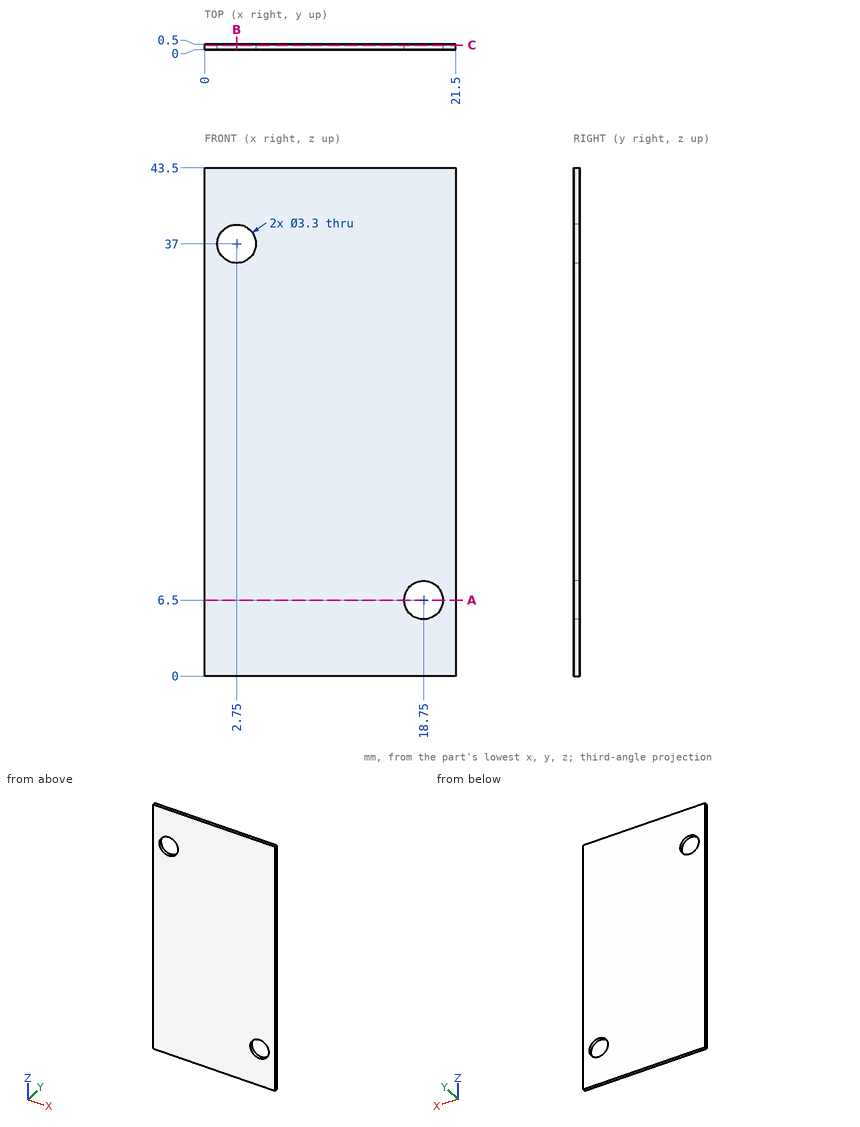
The drawing under review shows one solid part. Ordinate dimensions are in mm from its lowest x, y, z. Coordinates: 2 decimals unless noted, no trailing zeros. Write each loop counter-clockwise with the first axis right and the second up, starting at its lowest first coordinate (ties: lowest second). Pieces come first, ordered by that corner, then holes. Notation, with made-up numbers: (-3.5, -22.5) - (52.5, -22.5) arc R16 ccw to (52.5, 8.5) - close; hole circle Ø3 at (86.25, -4.5). An arc over 180 degrees is marked (long way). Put each result on its own line as item: value.
1. Wall thickness on probe 1 along Z at (x, y) = (2.75, 0.35); probe 2 along X at (y, z) = (0.1, 36.5); probe 3 along Z at (x, y) = (3.5, 0.3): over which ranges is each line inside the solid? List them lowest first.
Values found:
probe 1: 0 to 35.35, 38.65 to 43.5
probe 2: 0 to 1.18, 4.32 to 21.5
probe 3: 0 to 35.53, 38.47 to 43.5
2. Add section C-C, the plane y = 0.4. Give the boundary of the cut face in (x, z).
Values found:
outline: (0, 0) - (21.5, 0) - (21.5, 43.5) - (0, 43.5) - close; hole circle Ø3.3 at (2.75, 37); hole circle Ø3.3 at (18.75, 6.5)
3. Add section A-A, the plane z = 6.5. Give the boundary of the cut face in (x, y).
Values found:
outline: (0, 0) - (17.1, 0) - (17.1, 0.5) - (0, 0.5) - close; (20.4, 0) - (21.5, 0) - (21.5, 0.5) - (20.4, 0.5) - close
4. Add section B-B, the plane x = 2.75. Give the boundary of the cut face in (y, z).
Values found:
outline: (0, 0) - (0.5, 0) - (0.5, 35.35) - (0, 35.35) - close; (0, 38.65) - (0.5, 38.65) - (0.5, 43.5) - (0, 43.5) - close
